from build123d import *

# Parameters (mm, degrees)
F1_DEPTH  = 2
F3_DEPTH  = 7
F4_R      = 2.5
F4_W      = 5
F4_H      = 3
F5_DEPTH  = 5.5
F6_R      = 1.5
F7_DEPTH  = 1.8
F9_DEPTH  = 1.5
F10_SIZE  = 2
F12_DEPTH = 2
F13_SIZE  = 2


# Not quite as in the source:
# - a feature names something its author has since deleted; it is built from what else it names


with BuildPart() as f1:
    # F0 (on Top) → F1 (new body)
    with BuildSketch(Plane.XY):
        with BuildLine():
            Line((2.46, -15.24), (2.46, -2.54))
            Line((2.46, -2.54), (22.3642048012, -2.54))
            Line((22.3642048012, -2.54), (23.5517361372, -3.81))
            Line((23.5517361372, -3.81), (48.26, -3.81))
            ThreePointArc((48.26, -3.81), (50.8, -1.27), (48.26, 1.27))
            Line((48.26, 1.27), (31.75, 1.27))
            Line((31.75, 1.27), (31.75, 48.26))
            Line((31.75, 48.26), (43.18, 48.26))
            ThreePointArc((43.18, 48.26), (45.72, 50.8), (43.18, 53.34))
            Line((43.18, 53.34), (15.24, 53.34))
            ThreePointArc((15.24, 53.34), (12.7, 50.8), (15.24, 48.26))
            Line((15.24, 48.26), (26.67, 48.26))
            Line((26.67, 48.26), (26.67, 1.27))
            Line((26.67, 1.27), (11.8467498474, 1.27))
            Line((11.8467498474, 1.27), (10.6592185114, 2.54))
            Line((10.6592185114, 2.54), (0, 2.54))
            ThreePointArc((0, 2.54), (-1.7960512242, 1.7960512242), (-2.54, 0))
            Line((-2.54, 0), (-2.54, -15.24))
            Line((-2.54, -15.24), (2.46, -15.24))
        make_face()
    extrude(amount=F1_DEPTH)

    # F2 (on Top) → F3 (join)
    with BuildSketch(Plane.XY):
        Polygon((2.46, -18.24), (2.46, -15.24), (-2.54, -15.24), (-2.54, -10.24), (-5.54, -10.24), (-5.54, -18.24), align=None)
    extrude(amount=F3_DEPTH)

    # F4 (on Top) → F5 (join)
    with BuildSketch(Plane.XY):
        Circle(F4_R)
        with Locations((48.26, -1.27)):
            Circle(F4_R)
        with Locations((15.24, 50.8)):
            Circle(F4_R)
        with Locations((43.18, 50.8)):
            Circle(F4_R)
        with Locations((-0.04, -13.74)):
            Rectangle(F4_W, F4_H)
    extrude(amount=F5_DEPTH)

    # F6 (on face) → F7 (join)
    with BuildSketch(Plane.XY.offset(5.5)):
        Circle(F6_R)
        with Locations((48.26, -1.27)):
            Circle(F6_R)
        with Locations((15.24, 50.8)):
            Circle(F6_R)
        with Locations((43.18, 50.8)):
            Circle(F6_R)
    extrude(amount=F7_DEPTH)

    # F8 (on face) → F9 (cut)
    with BuildSketch(Plane.XY.offset(7)):
        Polygon((2.46, -15.24), (-2.54, -15.24), (-2.54, -10.24), (-2.84, -10.24), (-2.84, -15.54), (2.46, -15.54), align=None)
    extrude(amount=-F9_DEPTH, mode=Mode.SUBTRACT)

    # F10
    f10_edges = [f1.edges().sort_by_distance(p)[0] for p in [
        (31.75, 48.26, 1),
        (26.67, 48.26, 1),
        (26.67, 1.27, 1),
        (31.75, 1.27, 1),
        (2.46, -2.54, 1),
    ]]
    chamfer(f10_edges, length=F10_SIZE)

    # F11 (on Top) → F12 (join)
    with BuildSketch(Plane.XY):
        with BuildLine():
            ThreePointArc((37.5112494996, 23.515), (33.95, 24.765), (37.5112494996, 26.015))
            Line((37.5112494996, 26.015), (39.7496710384, 26.015))
            ThreePointArc((39.7496710384, 26.015), (35.95, 28.765), (32.1503289616, 26.015))
            ThreePointArc((32.1503289616, 26.015), (31.95, 24.765), (32.1503289616, 23.515))
            ThreePointArc((32.1503289616, 23.515), (35.95, 20.765), (39.7496710384, 23.515))
            Line((39.7496710384, 23.515), (37.5112494996, 23.515))
        make_face()
        with BuildLine():
            ThreePointArc((32.1503289616, 23.515), (31.95, 24.765), (32.1503289616, 26.015))
            Line((32.1503289616, 26.015), (31.75, 26.015))
            Line((31.75, 26.015), (31.75, 23.515))
            Line((31.75, 23.515), (32.1503289616, 23.515))
        make_face()
        with BuildLine():
            ThreePointArc((16.1096710384, 26.015), (12.31, 28.765), (8.5103289616, 26.015))
            Line((8.5103289616, 26.015), (10.7487505004, 26.015))
            ThreePointArc((10.7487505004, 26.015), (14.31, 24.765), (10.7487505004, 23.515))
            Line((10.7487505004, 23.515), (8.5103289616, 23.515))
            ThreePointArc((8.5103289616, 23.515), (12.31, 20.765), (16.1096710384, 23.515))
            ThreePointArc((16.1096710384, 23.515), (16.31, 24.765), (16.1096710384, 26.015))
        make_face()
        with BuildLine():
            Line((26.67, 26.015), (16.1096710384, 26.015))
            ThreePointArc((16.1096710384, 26.015), (16.31, 24.765), (16.1096710384, 23.515))
            Line((16.1096710384, 23.515), (26.67, 23.515))
            Line((26.67, 23.515), (26.67, 26.015))
        make_face()
    extrude(amount=F12_DEPTH)

    # F13
    f13_edges = [f1.edges().sort_by_distance(p)[0] for p in [
        (26.67, 23.515, 1),
        (26.67, 26.015, 1),
    ]]
    chamfer(f13_edges, length=F13_SIZE)


solid = f1.part
The listing builds one solid part. Answer for the finished solid, in the listing's coordinates (mm). A direction names the side the tool comes from. Round coordinates to 2 decimals unless told otherwise and drop trailing zeros. Write each loop counter-clockwise with the first axis right and the second up, starting at its lowest first coordinate (ties: lowest second). Pieces come first, ordered by that corner, then holes. Notation, with made-up numbers: (84.25, 69) - (126.25, 69) arc R13 cw to (126.25, 93) - close; hole circle Ø2 at (16.25, 40). An arc over 180 degrees is marked (long way). Use one line per item in the form item = value. Start each with the question number.
Item 1: A cutting plane is placed at D-D (y = -9). Write down the section's boundary in (x, z), plus the area to 4 significant figures.
Item 2: A tool of negligible diameter and unlimited length cuts with its end or side. For faces 4 (the cylindrical face through (49.69, -0.82, 6.39)), 5 (the flat face through (32.76, 2.26, 0.99)), 6 (the flat face through (10, 23.515, 1)), 7 (the cylindrical face through (36.02, 28.764, 0.986)), from which of +Z, -Z, +X, -X, +Y, -Y can it reach the whole face along a straight path? Write none if from no direction.
Item 3: A cutting plane is placed at B-B (z = 2.75). Write down the section's boundary in (x, y).
Item 4: Determine the mould class of faces 1 (the flat face through (25.66, 47.27, 0.99)), 2 (the flat face through (0, 0, 7.3)), 3 (the cylindrical face through (50.57, -2.23, 3.73)) for opening direction Y: +Y half, -Y half, draft (parallel to the pull), parting line (faces both ways), or undercut.
Item 5: Find the intervals of material crossed by line 1 (Y direction, x = 18, z = 1.5) (3 decimals); line 2 (Y direction, x = 12.31, z = 1) (3 decimals); line 3 (X direction, y = 27, z = 1.75) (3 decimals), in increasing order. Write a range as [from, to].
Item 6: Flat-ended cylindrical pins translate along their axes: pin 1 Ø1.6 at (y, z) = (34, 1) entering from -X; pin 2 Ø0.6 at (y, z) = (-11.5, 3) entering from +X; pin 3 Ø1.6 at (x, z) = (20.5, 1) entering from -Y. Find the tip coordinate at first contact, or state that the pin passes through.
Item 7: A cutting plane is placed at C-C (y = 6). Write down the section's boundary in (x, z), plus the area to 3 significant figures.
Item 8: A cutting plane is placed at A-A (x = 35.95). Write down the section's boundary in (y, z) (3 decimals), plus the area to 3 significant figures.
The answers:
q1.outline = (-2.54, 0) - (2.46, 0) - (2.46, 2) - (-2.54, 2) - close
q1.area = 10.00 mm^2
q2.face_4 = +Z
q2.face_5 = +Z, -Z, +X
q2.face_6 = +Z, -Z, -X
q2.face_7 = +Z, -Z
q3.outline = (-5.54, -18.24) - (2.46, -18.24) - (2.46, -12.24) - (-2.54, -12.24) - (-2.54, -10.24) - (-5.54, -10.24) - close; circle Ø5 at (0, 0); circle Ø5 at (15.24, 50.8); circle Ø5 at (43.18, 50.8); circle Ø5 at (48.26, -1.27)
q4.face_1 = undercut
q4.face_2 = draft
q4.face_3 = parting line
q5.line_1 = [-2.54, 1.27], [23.515, 26.015], [48.26, 53.34]
q5.line_2 = [-2.54, 1.27], [20.765, 22.765], [26.765, 28.765]
q5.line_3 = [8.993, 15.627], [25.655, 31.75], [32.633, 39.267]
q6.pin_1 = 26.67
q6.pin_2 = -2.54
q6.pin_3 = -2.54
q7.outline = (26.67, 0) - (31.75, 0) - (31.75, 2) - (26.67, 2) - close
q7.area = 10.2 mm^2
q8.outline = (-3.81, 0) - (1.27, 0) - (1.27, 2) - (-3.81, 2) - close; (20.765, 0) - (22.765, 0) - (22.765, 2) - (20.765, 2) - close; (26.765, 0) - (28.765, 0) - (28.765, 2) - (26.765, 2) - close; (48.26, 0) - (53.34, 0) - (53.34, 2) - (48.26, 2) - close
q8.area = 28.3 mm^2
